```python
from build123d import *

# Parameters (mm, degrees)
SKETCH1_W           = 107.5
SKETCH1_H           = 96
BOSS_EXTRUDE1_DEPTH = 5
SKETCH2_R           = 1.9
SKETCH2_R_2         = 11.5
SKETCH2_R_3         = 2.3
CUT_EXTRUDE3_DEPTH  = 5


with BuildPart() as part:
    # Sketch1 → Boss-Extrude1 (new body)
    with BuildSketch(Plane(origin=(0, 0, 0), x_dir=(1, 0, 0), z_dir=(0, 1, 0))):
        Rectangle(SKETCH1_W, SKETCH1_H)
    extrude(amount=BOSS_EXTRUDE1_DEPTH)

    # Sketch2 → Cut-Extrude3 (cut)
    with BuildSketch(Plane(origin=(0, 0, 0), x_dir=(1, 0, 0), z_dir=(0, 1, 0))):
        with Locations((-15.6, 15.6)):
            Circle(SKETCH2_R)
        with Locations((15.6, 15.6)):
            Circle(SKETCH2_R)
        with Locations((15.6, -15.6)):
            Circle(SKETCH2_R)
        with Locations((-15.6, -15.6)):
            Circle(SKETCH2_R)
        Circle(SKETCH2_R_2)
        with Locations((-43.255523212, -38.628188171)):
            Circle(SKETCH2_R_3)
        with Locations((43.42574654, 38.780201561)):
            Circle(SKETCH2_R_3)
        with Locations((-43.255523212, 38.628188171)):
            Circle(SKETCH2_R_3)
        with Locations((43.42574654, -38.780201561)):
            Circle(SKETCH2_R_3)
    extrude(amount=CUT_EXTRUDE3_DEPTH, mode=Mode.SUBTRACT)


solid = part.part
```
Build history of the part. All positions in model axes, mm. Coordinates: 2 decimals unless noted, no trailing zeros. Order: outer loops, then holes, each group sorted by start corner. A loop starts at its lowest first (then second) coordinate and runs counter-clockwise, first axis right, second up. Notation, with made-up numbers: M 13,-7 L 47,-7 A22 cw 47,1 Z; hole C -5.5,27 d6. An arc over 180 degrees is marked long. One line per question, with ' | ' between items. Start each with the question number.
1. Wall check: line 1 along X through (y, z) = (3.2, -15.6); line 2 along Z through (x, y) = (15.6, 2.5); line 3 along X through (y, z) = (3.6, -17). Give the ranges that are in metal, low to high. Write a range as [from, to].
2. Flat gauge pins, fed straight in: P1, Ø6, axis at x = 15.6, z = -15.6, coming from the +Y side; P2, Ø3.5, axis at x = -15.6, z = 15.6, coming from the -Y side. Where does each tip first touch, or does it go through?
3. Cut at D-D (x = -15.6). Write the cut outline in (y, z), plus the area to 3 significant figures.
4. Cut at B-B (z = 0). Write the cut outline in (x, y).
5. Cut at A-A (x = 0). Write the cut outline in (y, z), plus the area to 3 significant figures.
6. Mould opens along X. For faces 1 (the face through (-53.75, 2, 1)), 2 (the face through (-1.5, 2.5, -11.4)), 3 (the face through (-13, 5, -1)) say: +X half, -X half, draft (parallel to the pull), parting line (faces both ways), or undercut.
7. Cut at C-C (z = -15.6). Write the cut outline in (x, y).
The answers:
1) line 1: x = [-53.75, -17.5], [-13.7, 13.7], [17.5, 53.75] | line 2: z = [-48, -17.5], [-13.7, 13.7], [17.5, 48] | line 3: x = [-53.75, -16.88], [-14.32, 14.32], [16.88, 53.75]
2) P1: stops at y = 5 | P2: passes through
3) outline: M 0,-48 L 5,-48 L 5,-17.5 L 0,-17.5 Z; M 0,-13.7 L 5,-13.7 L 5,13.7 L 0,13.7 Z; M 0,17.5 L 5,17.5 L 5,48 L 0,48 Z | area: 442 mm2
4) outline: M -53.75,0 L -11.5,0 L -11.5,5 L -53.75,5 Z; M 11.5,0 L 53.75,0 L 53.75,5 L 11.5,5 Z
5) outline: M 0,-48 L 5,-48 L 5,-11.5 L 0,-11.5 Z; M 0,11.5 L 5,11.5 L 5,48 L 0,48 Z | area: 365 mm2
6) face 1: -X half | face 2: undercut | face 3: draft
7) outline: M -53.75,0 L -17.5,0 L -17.5,5 L -53.75,5 Z; M -13.7,0 L 13.7,0 L 13.7,5 L -13.7,5 Z; M 17.5,0 L 53.75,0 L 53.75,5 L 17.5,5 Z
